Geometry: final body of the model. Coordinates: model frame, mm. Face numbers are marked on the shaded views. A direction names the side the tool comes from. Round coordinates to 2 decimals unless told otherwise and drop trailing zeros. Return JSON: item names as keys, results as strings.
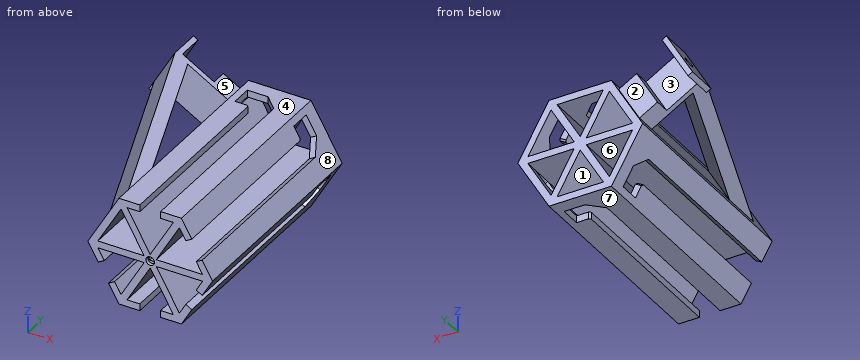
from build123d import *

# Parameters (mm, degrees)
SALIENTE_EXTRUIR1_DEPTH = 10
SALIENTE_EXTRUIR2_DEPTH = 170
CORTAR_EXTRUIR1_DEPTH   = 4
MATRIZC1_COUNT          = 5
MATRIZC1_ANGLE          = 240
CROQUIS4_W              = 24
CROQUIS4_H              = 12
SALIENTE_EXTRUIR3_DEPTH = 36
CROQUIS5_W              = 24
CROQUIS5_H              = 9
CORTAR_EXTRUIR2_DEPTH   = 24
CHAFL_N1_SIZE2          = 36
CHAFL_N1_SIZE           = 98.9091871
CORTAR_EXTRUIR3_DEPTH   = 24
CROQUIS7_W              = 30
CROQUIS7_H              = 18
CROQUIS7_R              = 3
SALIENTE_EXTRUIR4_DEPTH = 3
CROQUIS8_W              = 250
CROQUIS8_H              = 250
CORTAR_EXTRUIR4_DEPTH   = 84
CROQUIS9_R              = 2.5
CORTAR_EXTRUIR5_DEPTH   = 2
CORTAR_EXTRUIR6_DEPTH   = 7.9


with BuildPart() as part:
    # Croquis1 → Saliente-Extruir1 (new body)
    with BuildSketch(Plane(origin=(0, 0, 0), x_dir=(1, 0, 0), z_dir=(0, 1, 0))):
        Polygon((-12, 51.961524227), (-30, 51.961524227), (-39, 36.373066959), (-27, 15.588457268), (-51, 15.588457268), (-60, 0), (-51, -15.588457268), (-27, -15.588457268), (-39, -36.373066959), (-30, -51.961524227), (-12, -51.961524227), (0, -31.176914536), (12, -51.961524227), (30, -51.961524227), (39, -36.373066959), (27, -15.588457268), (51, -15.588457268), (60, 0), (51, 15.588457268), (27, 15.588457268), (39, 36.373066959), (30, 51.961524227), (12, 51.961524227), (0, 31.176914536), align=None)
    extrude(amount=SALIENTE_EXTRUIR1_DEPTH)

    # Croquis2 → Saliente-Extruir2 (add)
    # profile 1 of 2: a face of its own
    with BuildSketch(Plane(origin=(0, 10, 0), x_dir=(1, 0, 0), z_dir=(0, 1, 0))):
        Polygon((36, 0), (18, 31.176914536), (-18, 31.176914536), (-36, 0), (-18, -31.176914536), (18, -31.176914536), align=None)
        Polygon((15.690598923, 27.176914536), (-15.690598923, 27.176914536), (-31.381197846, 0), (-15.690598923, -27.176914536), (15.690598923, -27.176914536), (31.381197846, 0), align=None, mode=Mode.SUBTRACT)
    # profile 2 of 2: a face of its own
    with BuildSketch(Plane(origin=(0, 10, 0), x_dir=(1, 0, 0), z_dir=(0, 1, 0))):
        Polygon((-13.381197846, 27.176914536), (-15.690598923, 27.176914536), (-16.845299462, 25.176914536), (-3.464101615, 2), (-30.226497308, 2), (-31.381197846, 0), (-30.226497308, -2), (-3.464101615, -2), (-16.845299462, -25.176914536), (-15.690598923, -27.176914536), (-13.381197846, -27.176914536), (0, -4), (13.381197846, -27.176914536), (15.690598923, -27.176914536), (16.845299462, -25.176914536), (3.464101615, -2), (30.226497308, -2), (31.381197846, 0), (30.226497308, 2), (3.464101615, 2), (16.845299462, 25.176914536), (15.690598923, 27.176914536), (13.381197846, 27.176914536), (0, 4), align=None)
    extrude(amount=SALIENTE_EXTRUIR2_DEPTH)

    # Croquis3 → Cortar-Extruir1 (cut)
    with BuildSketch(Plane.XY.offset(31.176914536)):
        Polygon((-14, 172), (-2, 172), (6, 164), (6, 44), (-6, 44), (-6, 159.029437252), (-6.970562748, 160), (-14, 160), align=None)
    cortar_extruir1 = extrude(amount=-CORTAR_EXTRUIR1_DEPTH, mode=Mode.SUBTRACT)

    # MatrizC1: Cortar-Extruir1 ×5 about axis
    matrizc1_axis = Axis((0, 0, 0), (0, 1, 0))
    for i in range(1, MATRIZC1_COUNT):
        add(cortar_extruir1.rotate(matrizc1_axis, i * MATRIZC1_ANGLE / (MATRIZC1_COUNT - 1)), mode=Mode.SUBTRACT)

    # Croquis4 → Saliente-Extruir3 (add)
    with BuildSketch(Plane(origin=(-27, 0, 15.588457268), x_dir=(0.5000000000000002, 0, 0.8660254037844386), z_dir=(-0.8660254037844386, 0, 0.5000000000000002))):
        with Locations((0, 172)):
            Rectangle(CROQUIS4_W, CROQUIS4_H)
    extrude(amount=SALIENTE_EXTRUIR3_DEPTH)

    # Croquis5 → Cortar-Extruir2 (cut)
    with BuildSketch(Plane(origin=(-58.176914536, 0, 33.588457268), x_dir=(0.5000000000000003, 0, 0.8660254037844386), z_dir=(-0.8660254037844385, 0, 0.5000000000000002))):
        with Locations((0, 173.5)):
            Rectangle(CROQUIS5_W, CROQUIS5_H)
    extrude(amount=-CORTAR_EXTRUIR2_DEPTH, mode=Mode.SUBTRACT)

    # Chaflán1
    chafl_n1_edges = [part.edges().sort_by_distance(p)[0] for p in [
        (-27, 166, 15.588457268),
    ]]
    chafl_n1_side = [part.faces().sort_by_distance(p)[0] for p in [
        (-27, 165.28, 15.588457268),
    ]]
    chamfer(chafl_n1_edges, length=CHAFL_N1_SIZE - 0.0001, length2=CHAFL_N1_SIZE2 - 0.0001, reference=chafl_n1_side[0])  # a hair under: the kernel refuses the full size

    # Croquis6 → Cortar-Extruir3 (cut)
    with BuildSketch(Plane(origin=(-6, 0, -10.392304845), x_dir=(-0.8660254037844385, 0, 0.5000000000000003), z_dir=(-0.5000000000000003, 0, -0.8660254037844385))):
        Polygon((58.663492356, 166), (31.176914536, 90.481248101), (31.176914536, 166), align=None)
    extrude(amount=-CORTAR_EXTRUIR3_DEPTH, mode=Mode.SUBTRACT)

    # Croquis7 → Saliente-Extruir4 (add)
    with BuildSketch(Plane(origin=(-58.176914536, 0, 33.588457268), x_dir=(0.5000000000000003, 0, 0.8660254037844386), z_dir=(-0.8660254037844385, 0, 0.5000000000000002))):
        with Locations((-3, 175)):
            Rectangle(CROQUIS7_W, CROQUIS7_H)
        with Locations((-3, 175)):
            Circle(CROQUIS7_R, mode=Mode.SUBTRACT)
    extrude(amount=-SALIENTE_EXTRUIR4_DEPTH)

    # Croquis8 → Cortar-Extruir4 (cut)
    with BuildSketch(Plane(origin=(0, 54, 0), x_dir=(1, 0, 0), z_dir=(0, 1, 0))):
        Rectangle(CROQUIS8_W, CROQUIS8_H)
    extrude(amount=-CORTAR_EXTRUIR4_DEPTH, mode=Mode.SUBTRACT)

    # Croquis9 → Cortar-Extruir5 (cut)
    with BuildSketch(Plane.XZ.offset(-54)):
        with Locations(Location((0, 0, 0), (0, 0, 270))):
            Circle(CROQUIS9_R)
    extrude(amount=-CORTAR_EXTRUIR5_DEPTH, mode=Mode.SUBTRACT)

    # Croquis10 → Cortar-Extruir6 (cut)
    with BuildSketch(Plane.XZ.offset(-56)):
        with BuildLine():
            Line((1.528888485, 0.95), (-1.528888485, 0.95))
            ThreePointArc((-1.528888485, 0.95), (-1.8, 0), (-1.528888485, -0.95))
            Line((-1.528888485, -0.95), (1.528888485, -0.95))
            ThreePointArc((1.528888485, -0.95), (1.730895617, -0.493963929), (1.8, 0))
            ThreePointArc((1.8, 0), (1.730895617, 0.493963929), (1.528888485, 0.95))
        make_face()
    extrude(amount=-CORTAR_EXTRUIR6_DEPTH, mode=Mode.SUBTRACT)


solid = part.part
Q1. Reachability of the marked faces 1, 2, 3, 4 and 5 from +Z, -Z, +X, -X, +Y, -Y: full face, straight path, thin tool, end or side. Return the list, or none.
Determined:
{"face 1": "+Y, -Y", "face 2": "+Z, +Y", "face 3": "+Y", "face 4": "+Z, +X, +Y, -Y", "face 5": "+Z, +Y, -Y"}
Q2. Section query A-A (y = 98.5). State how many separate pieces and enclosed holes the cut face has, plus the area to 3 significant figures.
Determined:
{"separate pieces": "2", "enclosed holes": "1", "area": "1,470 mm^2"}
Q3. Material intervals for L1, parallel to X at y = 55, z = 0; L2, parallel to X at y = 94, z = 28; L3, parallel to Z at x = -21.5, y = 106, sorted ascending.
Determined:
{"L1": "x = -36 to -2.5, 2.5 to 36", "L2": "x = -31.14 to -24.5, -19.83 to -6, 6 to 19.83", "L3": "z = -25.11 to -19.34, -2 to 2, 17.11 to 25.11"}
Q4. Pin query (flat end, axial travel): pin 1 (2 mm diameter, centred on x = -21.5, z = -23.5, fed in from +Y); pin 2 (1 mm diameter, centred on y = 84.5, z = 20.5, fed in from +X); pin 3 (0.7 mm diameter, centred on x = 13.5, y = 164, fed in from -Z). Return the tip coordinate at first contact, or that it passes through.
Determined:
{"pin 1": "stops at y = 180", "pin 2": "stops at x = 24", "pin 3": "stops at z = -27.18"}
Q5. Pull-direction query (X, two-part tool) for the marked faces 6, 7 and 8; classes: pulls with the +X half, pulls with the -X half, needs draft (parallel to the pull), parting line crosses it, or undercut.
Determined:
{"face 6": "undercut", "face 7": "needs draft", "face 8": "pulls with the +X half"}
